from build123d import *

# Parameters (mm, degrees)
F0_W     = 50
F0_H     = 45
F1_DEPTH = 20
F2_W     = 40
F2_H     = 80
F3_DEPTH = 20


with BuildPart() as f1:
    # F0 (on Front) → F1 (new body)
    with BuildSketch(Plane.XZ):
        with Locations((0, 22.5)):
            Rectangle(F0_W, F0_H)
    extrude(amount=F1_DEPTH)

    # F2 (on Front) → F3 (cut)
    with BuildSketch(Plane.XZ):
        Rectangle(F2_W, F2_H)
    extrude(amount=F3_DEPTH, mode=Mode.SUBTRACT)


solid = f1.part
Work out the finished part from the listing and answer in its coordinate system (mm). A direction names the side the tool comes from. Give positions to 0.01 mm unless a question says otherwise; leave off trailing zeros. Loops run counter-clockwise (first coordinate to the right, second up) from the corner with the lowest first, then second, coordinate; pieces in that order, holes last. Notation, with made-up numbers: M 24.5,44.25 L 49.5,44.25 A23 cw 49.5,69.25 Z; hole C 1.5,48.25 d2. An arc over 180 degrees is marked long. Use CSV: the item, a comma, the result in double quotes.
1) Find section B-B on y = -6. Write down the section's boundary in (x, z), plus the area to 3 significant figures.
Answer:
outline,"M -25,0 L -20,0 L -20,40 L 20,40 L 20,0 L 25,0 L 25,45 L -25,45 Z"
area,"650 mm^2"
2) Find section A-A on z = 38. Write down the section's boundary in (x, y), plus the area to 3 significant figures.
Answer:
outline,"M -25,-20 L -20,-20 L -20,0 L -25,0 Z; M 20,-20 L 25,-20 L 25,0 L 20,0 Z"
area,"200 mm^2"
3) Consider L1, parallel to X at y = -7.5, z = 5.5; L2, parallel to Z at x = -15.5, y = -16.25. Determine where each line is inside the solid, lowest interval first.
Answer:
L1,"-25 to -20, 20 to 25"
L2,"40 to 45"
4) Given P1, Ø3, axis at x = -6.5, y = -5, coming from the -Z side, flat-ended and moving along its own axis, determine where the tip first touches the part or whether it passes through.
Answer:
P1,"z = 40"
5) Find section C-C on x = 10. Write down the section's boundary in (y, z).
Answer:
outline,"M -20,40 L 0,40 L 0,45 L -20,45 Z"
6) Which of the six approach directions +Z, -Z, +X, -X, +Y, -Y give full straight-line access (tool end or side, diameter ignored) to faces 1 (the flat face through (0, -10, 40)), 2 (the flat face through (-23, -10, 0))?
Answer:
face 1,"-Z, +Y, -Y"
face 2,"-Z, +X, -X, +Y, -Y"
7) Determine the mould class of faces 3 (the flat face through (22, -10, 0)), 4 (the flat face through (-25, -10, 22)), 5 (the flat face through (-20, -10, 20)) for opening direction X: released by +X, released by -X, zero draft, split by the parting line, or undercut.
Answer:
face 3,"zero draft"
face 4,"released by -X"
face 5,"undercut"
